Source: CAD feature listing. Evaluate the final solid. Frame: model axes, mm. A direction names the side the tool comes from. Give positions to 0.01 mm unless a question says otherwise; leave off trailing zeros. Loops run counter-clockwise (first coordinate to the right, second up) from the corner with the lowest first, then second, coordinate; pieces in that order, holes last. Notation, with made-up numbers: M 19,42.25 L 45,42.25 A24 ccw 45,79.25 Z; hole C 11.5,69.5 d6. An arc over 180 degrees is marked long. Answer in a Markdown table with one row per item.
```python
from build123d import *

# Parameters (mm, degrees)
SKETCH1_R           = 1.778
SKETCH1_R_2         = 1.5875
BOSS_EXTRUDE1_DEPTH = 3.175
SKETCH2_R           = 4.7625
SKETCH2_R_2         = 1.5875
BOSS_EXTRUDE2_DEPTH = 6.35
SKETCH3_R           = 3.302
CUT_EXTRUDE1_DEPTH  = 3.175
FILLET1_R           = 1.5875


with BuildPart() as part:
    # Sketch1 → Boss-Extrude1 (new body)
    with BuildSketch(Plane(origin=(0, 0, 0), x_dir=(1, 0, 0), z_dir=(0, 1, 0))):
        with BuildLine():
            Line((6.35, 15.367), (6.35, -15.367))
            ThreePointArc((6.35, -15.367), (0, -21.717), (-6.35, -15.367))
            Line((-6.35, -15.367), (-6.35, 15.367))
            ThreePointArc((-6.35, 15.367), (0, 21.717), (6.35, 15.367))
        make_face()
        with Locations(Location((0, 15.367, 0), (0, 0, 270))):
            Circle(SKETCH1_R, mode=Mode.SUBTRACT)
        with Locations(Location((0, -15.367, 0), (0, 0, 270))):
            Circle(SKETCH1_R, mode=Mode.SUBTRACT)
        with Locations(Location((0, 0, 0), (0, 0, 270))):
            Circle(SKETCH1_R_2, mode=Mode.SUBTRACT)
    extrude(amount=BOSS_EXTRUDE1_DEPTH)

    # Sketch2 → Boss-Extrude2 (add)
    with BuildSketch(Plane(origin=(0, 3.175, 0), x_dir=(1, 0, 0), z_dir=(0, 1, 0))):
        with Locations(Location((0, 0, 0), (0, 0, 270))):
            Circle(SKETCH2_R)
        with Locations(Location((0, 0, 0), (0, 0, 270))):
            Circle(SKETCH2_R_2, mode=Mode.SUBTRACT)
    extrude(amount=BOSS_EXTRUDE2_DEPTH)

    # Sketch3 → Cut-Extrude1 (cut)
    with BuildSketch(Plane(origin=(0, 9.525, 0), x_dir=(1, 0, 0), z_dir=(0, 1, 0))):
        with Locations(Location((0, 0, 0), (0, 0, 270))):
            Circle(SKETCH3_R)
    extrude(amount=-CUT_EXTRUDE1_DEPTH, mode=Mode.SUBTRACT)

    # Fillet1
    fillet1_edges = [part.edges().sort_by_distance(p)[0] for p in [
        (0, 3.175, -4.7625),
    ]]
    fillet(fillet1_edges, radius=FILLET1_R - 0.0001)  # a hair under: the kernel refuses the full size


solid = part.part
```
1) Material intervals for L1, parallel to X at y = 3, z = 0; L2, parallel to Y at x = -5.25, z = -8.5 (3 decimals); L3, parallel to X at y = 8.05, z = 0, sorted ascending.
Reply:
| item | result |
|---|---|
| L1 | x = -6.35 to -1.59, 1.59 to 6.35 |
| L2 | y = 0 to 3.175 |
| L3 | x = -4.76 to -3.3, 3.3 to 4.76 |
2) Section D-D, the plane y = 7.75. Return loops of the section in (x, z) (1 decimal), then the cut area to 3 significant figures.
Reply:
| item | result |
|---|---|
| outline | C 0,0 d9.5; hole C 0,0 d6.6 |
| area | 37.0 mm² |
3) Set-up query: faces 4 (the cylindrical face through (-0.681, 1.565, -13.725)), 5 (the cylindrical face through (0.99, 7.96, 3.15)). Return all of +Z, -Z, +X, -X, +Y, -Y with unobstructed straight access to the full face (end or side cutting, diameter ignored); none if empty.
Reply:
| item | result |
|---|---|
| face 4 | +Y, -Y |
| face 5 | +Y |
4) Pin query (flat end, axial travel): pin 1 Ø6 at (x, z) = (4.5, -17.5) entering from +Y (3 decimals); pin 2 Ø4 at (x, z) = (0, 0) entering from +Y. Return the tip coordinate at first contact, or that it passes through.
Reply:
| item | result |
|---|---|
| pin 1 | stops at y = 3.175 |
| pin 2 | stops at y = 6.35 |
5) Section B-B, the plane x = 0. Count the separate pieces of the cut face and the enclosed holes in it, then the cut area to 3 significant figures.
Reply:
| item | result |
|---|---|
| separate pieces | 4 |
| enclosed holes | 0 |
| area | 136 mm² |
6) Pull-direction query (X, two-part tool) for faces 1 (the cylindrical face through (-1.082, 1.565, 13.956)), 2 (the flat face through (-6.35, 2, 0)), 3 (the cylindrical face through (-0.14, 1.565, -21.715)); classes: released by +X, released by -X, zero draft, split by the parting line, or undercut.
Reply:
| item | result |
|---|---|
| face 1 | undercut |
| face 2 | released by -X |
| face 3 | split by the parting line |
